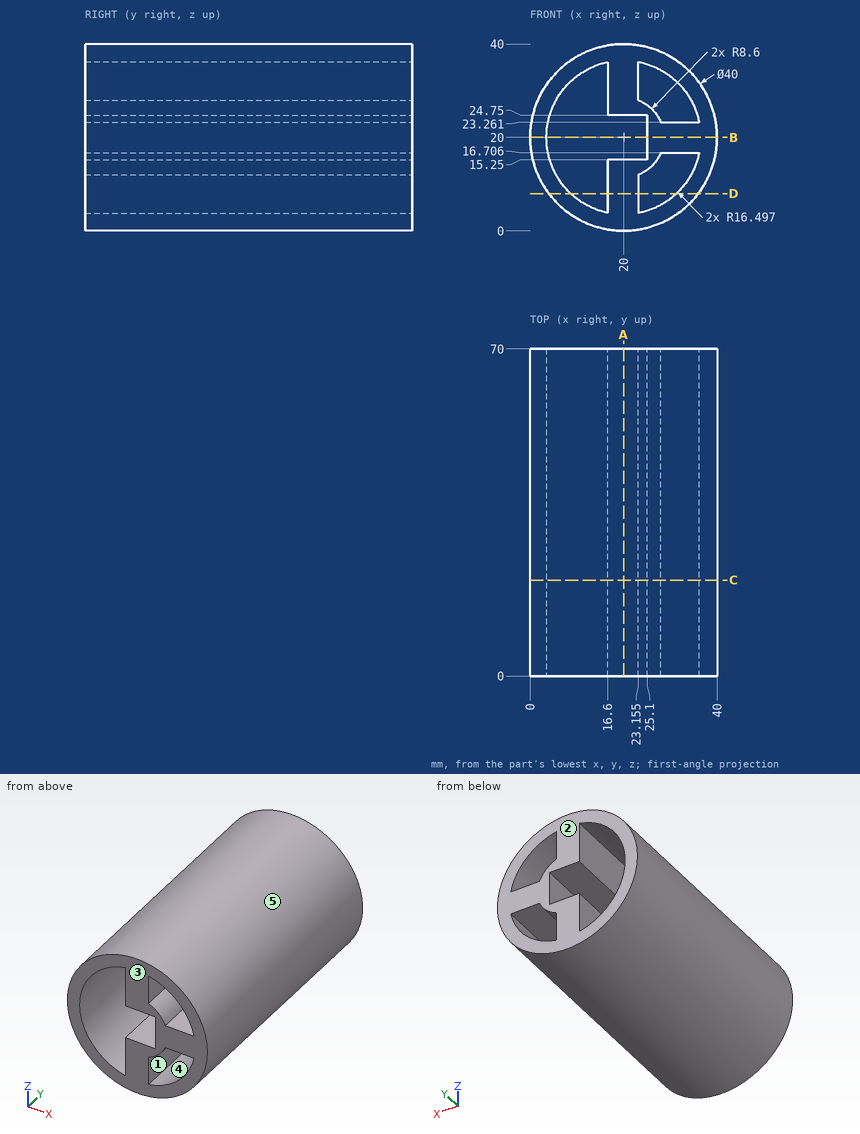
Part print with two shaded views. Sizes in mm from the minimum x, y, z corner. A direction names the side the tool comes from. Round coordinates to 2 decimals unless told otherwise and drop trailing zeros. Loops run counter-clockwise (first coordinate to the right, second up) from the corner with the lowest first, then second, coordinate; pieces in that order, holes last. Notation, with made-up numbers: (77.25, 12) - (121.25, 12) arc R27 cw to (121.25, 37) - close; hole circle Ø8 at (-10.75, -32.75). An arc over 180 degrees is marked (long way). Answer as a JSON object with one key per item and string values.
Item 1: Tool access for the marked faces 1 and 2: list every direction of +Z, -Z, +X, -X, +Y, -Y with a clear straight run to the whole face (end or side of a thin tool).
Output:
{"face 1": "+Y, -Y", "face 2": "+Z, -Z, +X, -X, +Y"}
Item 2: Band-saw the part on C-C on y = 20.5. State how many separate pieces and enclosed holes the cut face has.
Output:
{"separate pieces": "1", "enclosed holes": "3"}
Item 3: Wall check: L1, parallel to Z at x = 34, y = 18.5 (1 decimal); L2, parallel to X at y = 60.5, z = 14.5 (1 decimal); L3, parallel to Z at x = 20, y = 18. Give the ranges that are in metal, low to high.
Output:
{"L1": "5.7 to 11.3, 16.7 to 23.3, 28.7 to 34.3", "L2": "0.8 to 4.4, 16.6 to 26.6, 35.6 to 39.2", "L3": "0 to 15.25, 24.75 to 40"}
Item 4: Band-saw the part on D-D on z = 8. List the corners of the cut face in (x, y) (1 decimal).
Output:
{"outline": "(4, 0) - (8.7, 0) - (8.7, 70) - (4, 70) - close; (16.6, 0) - (23.2, 0) - (23.2, 70) - (16.6, 70) - close; (31.3, 0) - (36, 0) - (36, 70) - (31.3, 70) - close"}
Item 5: Band-saw the part on B-B on z = 20. List the corners of the cut face in (x, y).
Output:
{"outline": "(0, 0) - (3.5, 0) - (3.5, 70) - (0, 70) - close; (25.1, 0) - (40, 0) - (40, 70) - (25.1, 70) - close"}
Item 6: Pull direction Z, two halves, no side cores. Call the marked faces 3, 4 and 5: pulls with the +Z half, pulls with the -Z half, needs draft (parallel to the pull), parting line crosses it, or undercut.
Output:
{"face 3": "needs draft", "face 4": "undercut", "face 5": "parting line crosses it"}
Item 7: Pin check, flat tips, straight feed: pin 1 (1 mm diameter, centred on y = 56, z = 5, fed in from +X) (1 decimal); pin 2 (3 mm diameter, centred on x = 26, z = 18.5, fed in from -Y); pin 3 (2.5 mm diameter, centred on x = 33, y = 50, fed in from +Z) (1 decimal); pin 4 (3 mm diameter, centred on x = 10.5, y = 47, fed in from -Z). Stop position of each tip, or through.
Output:
{"pin 1": "x = 33.8", "pin 2": "y = 0", "pin 3": "z = 36.2", "pin 4": "z = 1.67"}
Item 8: Band-saw the part on A-A on x = 20. List the corners of the cut face in (y, z).
Output:
{"outline": "(0, 0) - (70, 0) - (70, 15.25) - (0, 15.25) - close; (0, 24.75) - (70, 24.75) - (70, 40) - (0, 40) - close"}
